from build123d import *

# Parameters (mm, degrees)
PAD_DEPTH    = 0.7
PAD001_DEPTH = 61
FILLET_R     = 1
FILLET001_R  = 0.3


with BuildPart() as part:
    # Sketch004 (on DatumPlane) → Pad (new body)
    with BuildSketch(Plane(origin=(0, 0, 38.1), x_dir=(0, 1, 0), z_dir=(0, 0, 1))):
        with BuildLine():
            ThreePointArc((-58.799235, -0.3), (0, -58.8), (58.799235, -0.3))
            Line((58.799235, -0.3), (-58.799235, -0.3))
        make_face()
    extrude(amount=PAD_DEPTH)

    # Sketch005 (on DatumPlane) → Pad001 (join, symmetric)
    with BuildSketch(Plane(origin=(0, 0, 0), x_dir=(-1, 0, 0), z_dir=(0, 1, 0))):
        with BuildLine():
            ThreePointArc((-4.766352, 38.8), (-3, 36.2), (-1.233648, 38.8))
            Line((-4.766352, 38.8), (-1.233648, 38.8))
        make_face()
    extrude(amount=PAD001_DEPTH, both=True)

    # Fillet
    fillet_edges = [part.edges().sort_by_distance(p)[0] for p in [
        (3, -61, 36.2),
        (3, 61, 36.2),
    ]]
    fillet(fillet_edges, radius=FILLET_R)

    # Fillet001
    fillet001_edges = [part.edges().sort_by_distance(p)[0] for p in [
        (0.3, 0, 38.8),
    ]]
    fillet(fillet001_edges, radius=FILLET001_R)


solid = part.part
Input: part model. Units: mm. Frame: model coordinates. A direction names the side the tool comes from. Round coordinates to 2 decimals unless told otherwise and drop trailing zeros. Order: outer loops, then holes, each group sorted by start corner. A loop starts at its lowest first (then second) coordinate and runs counter-clockwise, first axis right, second up.
1. Set-up query: faces 1 (the face through (24, 1, 38.8)), 2 (the face through (25, -1, 38.1)). Return all of +Z, -Z, +X, -X, +Y, -Y with unobstructed straight access to the full face (end or side cutting, diameter ignored); none if empty.
The answers:
face 1: +Z, +X, -X, +Y, -Y
face 2: -Z, +X, +Y, -Y
2. Pin query (flat end, axial travel): P1, Ø3, axis at x = 18, y = 19, coming from the -Z side; P2, Ø1.5, axis at x = 19.5, z = 36.5, coming from the +Y side. Return the tip coordinate at first contact, or that it passes through.
The answers:
P1: stops at z = 38.1
P2: passes through
3. Cut plane B-B, the plane x = 9.5. Output: boundary loops of the cut face in (y, z), then the cut area to 3 significant figures.
The answers:
outline: (-58.03, 38.1) - (58.03, 38.1) - (58.03, 38.8) - (-58.03, 38.8) - close
area: 81.2 mm2
4. Material intervals for line 1 (Z direction, x = 25.5, y = -30); line 2 (X direction, y = 2, z = 37.25); line 3 (Y direction, x = 5, z = 38.6), sorted ascending.
The answers:
line 1: z = 38.1 to 38.8
line 2: x = 1.3 to 4.7
line 3: y = -58.59 to 58.59
5. Cut plane C-C, the plane y = -26.5. Output: boundary loops of the cut face in (x, z), then the cut area to 3 significant figures.
The answers:
outline: (0.3, 38.1) - (1.1, 38.1) arc R1.9 ccw to (4.9, 38.1) - (52.49, 38.1) - (52.49, 38.8) - (0.6, 38.8) arc R0.3 ccw to (0.3, 38.5) - close
area: 42.2 mm2
6. Cut plane A-A, the plane y = 36.5. Output: boundary loops of the cut face in (x, z).
The answers:
outline: (0.3, 38.1) - (1.1, 38.1) arc R1.9 ccw to (4.9, 38.1) - (46.1, 38.1) - (46.1, 38.8) - (0.6, 38.8) arc R0.3 ccw to (0.3, 38.5) - close
